Part model, mm, in its own coordinate system. A direction names the side the tool comes from. Round coordinates to 2 decimals unless told otherwise and drop trailing zeros. Write each loop counter-clockwise with the first axis right and the second up, starting at its lowest first coordinate (ties: lowest second). Pieces come first, ordered by that corner, then holes. Notation, with made-up numbers: (78.25, -30) -> (116.25, -30) arc R29 cw to (116.25, 2) -> close; hole circle Ø9 at (28, 71). An arc over 180 degrees is marked (long way). Return JSON: item names as keys, results as strings. Group by question number.
(1) Drill centre lines: L1, parallel to X at y = -8, z = -20; L2, parallel to Z at x = 4.5, y = 0; L3, parallel to Z at x = -23.2, y = 0.7. Where is each one in solid material? Low to high. Write a range as from..to.
(2) Mould opens along X. For faces 1 (the flat face through (-6.627, -7, -21)), 2 (the flat face through (11.38, 0.52, 11.25)), 3 (the flat face through (-17, -5, -23.3)) say: +X half, -X half, draft (parallel to the pull), parting line (faces both ways), or undercut.
(3) Saw through at D-D (x = 10). List the corners of the cut face in (y, z).
(4) Saw through at B-B (x = 18). List the corners of the cut face in (y, z).
(5) Saw through at A-A (z = -29.5). List the corners of the cut face in (x, y).
(6) Drop flat-ended pins along their axis: pin 1 Ø2 at (x, y) = (-13, -7) entering from -Z; pin 2 Ø8 at (y, z) = (-8, -28) entering from -X; pin 3 Ø0.9 at (y, z) = (0, -36.5) entering from -X; pin 4 Ø1.5 at (x, y) = (-3, 0.5) entering from -Z. Give the stop position or say it passes through.
(7) Saw through at C-C (y = -12). List the corners of the cut face in (x, z).
(8) Tool access for faces 4 (the flat face through (16, 1, 0)), 5 (the flat face through (-12.393, -6.916, -12.234)), 6 (the flat face through (-27.154, 0.521, 24.024)), 7 (the cylindrical face through (-23.28, -10.13, -11.81)), 8 (the flat face through (-27.2, -6.9, 3.7)): list every direction of +Z, -Z, +X, -X, +Y, -Y with a clear straight run to the whole face (end or side of a thin tool).
from build123d import *

# Parameters (mm, degrees)
SKETCH_R           = 2.3
SKETCH_R_2         = 1
SKETCH_R_3         = 1.2
SKETCH_W           = 13
SKETCH_H           = 23.6
PAD_DEPTH          = 3
PAD005002_DEPTH    = 12
SKETCH002_R        = 2.15
POCKET_DEPTH       = 24
SKETCH003_R        = 2.15
POCKET002002_DEPTH = 7
POCKET002003_DEPTH = 3.001


with BuildPart() as part:
    # Sketch → Pad (new body)
    with BuildSketch(Plane.XZ):
        Polygon((-26.07868, 25.1), (11.672078, 25.1), (24.4, 12.372078), (24.4, -23.3), (24.4, -42.5), (16.9, -50), (-0.551549, -50), (-2.672869, -47.87868), (-2.672869, -28.369956), (-7.742825, -23.3), (-28.2, -23.3), (-28.2, 22.97868), align=None)
        with Locations((-23.2, 20.1)):
            Circle(SKETCH_R, mode=Mode.SUBTRACT)
        with Locations((19.4, -18.3)):
            Circle(SKETCH_R, mode=Mode.SUBTRACT)
        with Locations((10.01639, -19.647283)):
            Circle(SKETCH_R_2, mode=Mode.SUBTRACT)
        with Locations((10, -46.85)):
            Circle(SKETCH_R_3, mode=Mode.SUBTRACT)
        Polygon((16, 6.627417), (6.627417, 16), (-6.627417, 16), (-16, 6.627417), (-16, -6.627417), (-6.627417, -16), (6.627417, -16), (16, -6.627417), align=None, mode=Mode.SUBTRACT)
        with Locations((10, -33.2)):
            Rectangle(SKETCH_W, SKETCH_H, mode=Mode.SUBTRACT)
    extrude(amount=PAD_DEPTH)

    # Sketch001 (on Face30 of Pad) → Pad005002 (join)
    with BuildSketch(Plane.XZ.offset(3)):
        Polygon((-26.07868, 4.82132), (-20.12132, 4.82132), (-18, 2.7), (-18, -6.627417), (-6.627417, -18), (-6.627417, -23.3), (-28.2, -23.3), (-28.2, 2.7), align=None)
    extrude(amount=PAD005002_DEPTH)

    # Sketch002 (on Face38 of Pad005002) → Pocket (cut)
    with BuildSketch(Plane(origin=(0, 0, -24), x_dir=(1, 0, 0), z_dir=(0, 0, -1))):
        with Locations((-23, 10)):
            Circle(SKETCH002_R)
    extrude(amount=-POCKET_DEPTH, mode=Mode.SUBTRACT)

    # Sketch003 (on Face38 of Pad005002) → Pocket002002 (cut)
    with BuildSketch(Plane(origin=(0, 0, -24), x_dir=(1, 0, 0), z_dir=(0, 0, -1))):
        with Locations((-12, 10)):
            Circle(SKETCH003_R)
    extrude(amount=-POCKET002002_DEPTH, mode=Mode.SUBTRACT)

    # Sketch004 (on Face5 of Pocket002002) → Pocket002003 (cut, through all)
    with BuildSketch(Plane.XZ.offset(3)):
        Polygon((12.5, -43.35), (7.5, -43.35), (7.5, -46.35), (8, -46.85), (10, -46.85), (12, -46.85), (12.5, -46.35), align=None)
    extrude(amount=-POCKET002003_DEPTH, mode=Mode.SUBTRACT)


with BuildPart() as part_1:
    # Body placement: moved
    add(part.part.moved(Location((0, 2, 0))))


solid = part_1.part
Computed values:
{
 "1": {"L1": "-28.2..-25.15, -20.85..-14.15, -9.85..-6.63", "L2": "-50..-45, -21.4..-16, 16..25.1", "L3": "-23.3..17.8, 22.4..25.1"},
 "2": {"face 1": "+X half", "face 2": "undercut", "face 3": "draft"},
 "3": {"outline": "(-1, -50) -> (2, -50) -> (2, -48.05) -> (-1, -48.05) -> close; (-1, -21.4) -> (2, -21.4) -> (2, -20.65) -> (-1, -20.65) -> close; (-1, -18.65) -> (2, -18.65) -> (2, -12.63) -> (-1, -12.63) -> close; (-1, 12.63) -> (2, 12.63) -> (2, 25.1) -> (-1, 25.1) -> close"},
 "4": {"outline": "(-1, -48.9) -> (2, -48.9) -> (2, -20.12) -> (-1, -20.12) -> close; (-1, -16.48) -> (2, -16.48) -> (2, 18.77) -> (-1, 18.77) -> close"},
 "5": {"outline": "(-2.67, -1) -> (3.5, -1) -> (3.5, 2) -> (-2.67, 2) -> close; (16.5, -1) -> (24.4, -1) -> (24.4, 2) -> (16.5, 2) -> close"},
 "6": {"pin 1": "z = -23.3", "pin 2": "through", "pin 3": "x = -2.67", "pin 4": "z = -48.3"},
 "7": {"outline": "(-28.2, -23.3) -> (-6.63, -23.3) -> (-6.63, -18) -> (-18, -6.63) -> (-18, 2.7) -> (-20.12, 4.82) -> (-26.08, 4.82) -> (-28.2, 2.7) -> close"},
 "8": {"face 4": "+Y, -Y", "face 5": "+Z, +X, -Y", "face 6": "+Z, -X, +Y, -Y", "face 7": "-Z", "face 8": "+Z, -X, -Y"}
}
